Answer from the drawing. Dimensions are ordinates in mm from the lowest x, y and z of the part. A direction names the side the tool comes from. Give positions to 0.01 mm unless a question says otherwise; leave off trailing zeros. Order: outer loops, then holes, each group sorted by start corner. A loop starts at its lowest first (then second) coordinate and runs counter-clockwise, first axis right, second up.
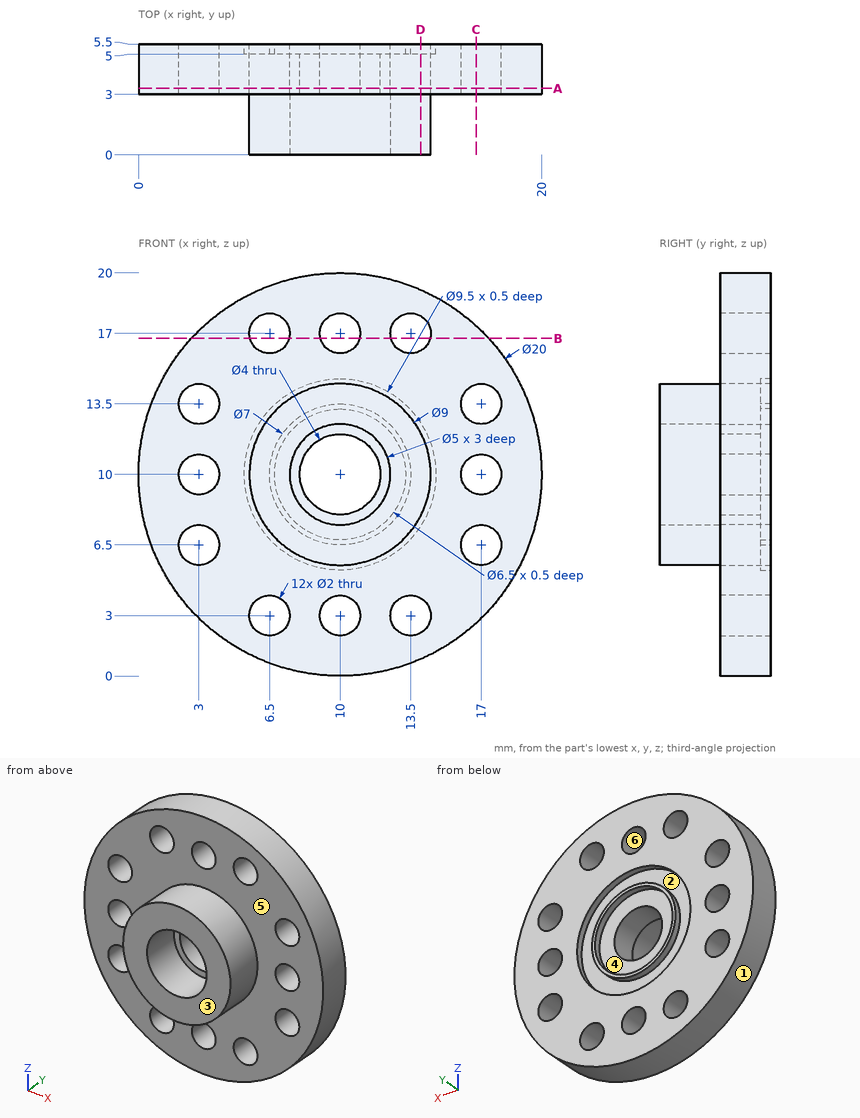
1) The part is cut by section C-C on x = 16.75. Determine the outline of the cut face in (y, z), and give its area (3 significant figures).
Final values:
outline: (3, 2.62) - (5.5, 2.62) - (5.5, 5.53) - (3, 5.53) - close; (3, 7.47) - (5.5, 7.47) - (5.5, 9.03) - (3, 9.03) - close; (3, 10.97) - (5.5, 10.97) - (5.5, 12.53) - (3, 12.53) - close; (3, 14.47) - (5.5, 14.47) - (5.5, 17.38) - (3, 17.38) - close
area: 22.4 mm2
2) The part is cut by section D-D on x = 14. Determine the outline of the cut face in (y, z), and give its area (3 significant figures).
Final values:
outline: (0, 7.94) - (3, 7.94) - (3, 3.87) - (5.5, 3.87) - (5.5, 7.44) - (5, 7.44) - (5, 12.56) - (5.5, 12.56) - (5.5, 16.13) - (3, 16.13) - (3, 12.06) - (0, 12.06) - close; (3, 0.83) - (5.5, 0.83) - (5.5, 2.13) - (3, 2.13) - close; (3, 17.87) - (5.5, 17.87) - (5.5, 19.17) - (3, 19.17) - close
area: 47.0 mm2
3) The part is cut by section A-A on y = 3.3. Count the separate pieces of the cut face and the enclosed holes in it, and give its area (3 significant figures).
Final values:
separate pieces: 1
enclosed holes: 13
area: 264 mm2
4) Given pin 1 (3 mm diameter, centred on y = 0.5, z = 10, fed in from +X); pin 2 (3 mm diameter, centred on x = 17, z = 10, fed in from -Y); pin 3 (3 mm diameter, centred on y = 3, z = 13, fed in from +X), each flat-ended and moving along its own axis, determine where each tip first touches the part or whether it passes through.
Final values:
pin 1: stops at x = 14.5
pin 2: stops at y = 3
pin 3: stops at x = 19.89
5) A tool of negligible diameter and unlimited length cuts with its end or side. For the marked faces 4, 5 and 6, from which of +Z, -Z, +X, -X, +Y, -Y can it reach the whole face along a straight path? Write none if from no direction.
Final values:
face 4: +Y
face 5: -Y
face 6: +Y, -Y
6) For a pull along X with two mould halves and no side action, classify the marked faces 1, 2 and 3 as released by +X, released by -X, zero draft, split by the parting line, or undercut.
Final values:
face 1: split by the parting line
face 2: undercut
face 3: zero draft
7) The part is cut by section B-B on z = 16.75. Determine the outline of the cut face in (x, y).
Final values:
outline: (2.62, 3) - (5.53, 3) - (5.53, 5.5) - (2.62, 5.5) - close; (7.47, 3) - (9.03, 3) - (9.03, 5.5) - (7.47, 5.5) - close; (10.97, 3) - (12.53, 3) - (12.53, 5.5) - (10.97, 5.5) - close; (14.47, 3) - (17.38, 3) - (17.38, 5.5) - (14.47, 5.5) - close
8) Consider L1, parallel to X at y = 4.1, z = 10; L2, parallel to X at y = 5.3, z = 10; L3, parallel to X at y = 4.6, z = 3. Determine where each line is inside the solid, lowest interval first.
Final values:
L1: x = 0 to 2, 4 to 8, 12 to 16, 18 to 20
L2: x = 0 to 2, 4 to 5.25, 6.5 to 6.75, 13.25 to 13.5, 14.75 to 16, 18 to 20
L3: x = 2.86 to 5.5, 7.5 to 9, 11 to 12.5, 14.5 to 17.14
